Here's the drawing with two shaded views (mm, measured from the low corner). I have some questions. A direction names the side the tool comes from. Give positions to 0.01 mm unless a question says otherwise; leave off trailing zeros. Write each loop counter-clockwise with the first axis right and the second up, starting at its lowest first coordinate (ties: lowest second). Pieces come first, ordered by that corner, then holes. Notation, with made-up numbers: (58.5, -6.75) -> (100.5, -6.75) arc R26 cw to (100.5, 13.25) -> close; hole circle Ø7 at (31, 10). An arc over 180 degrees is marked (long way). One line per item, written item: value.
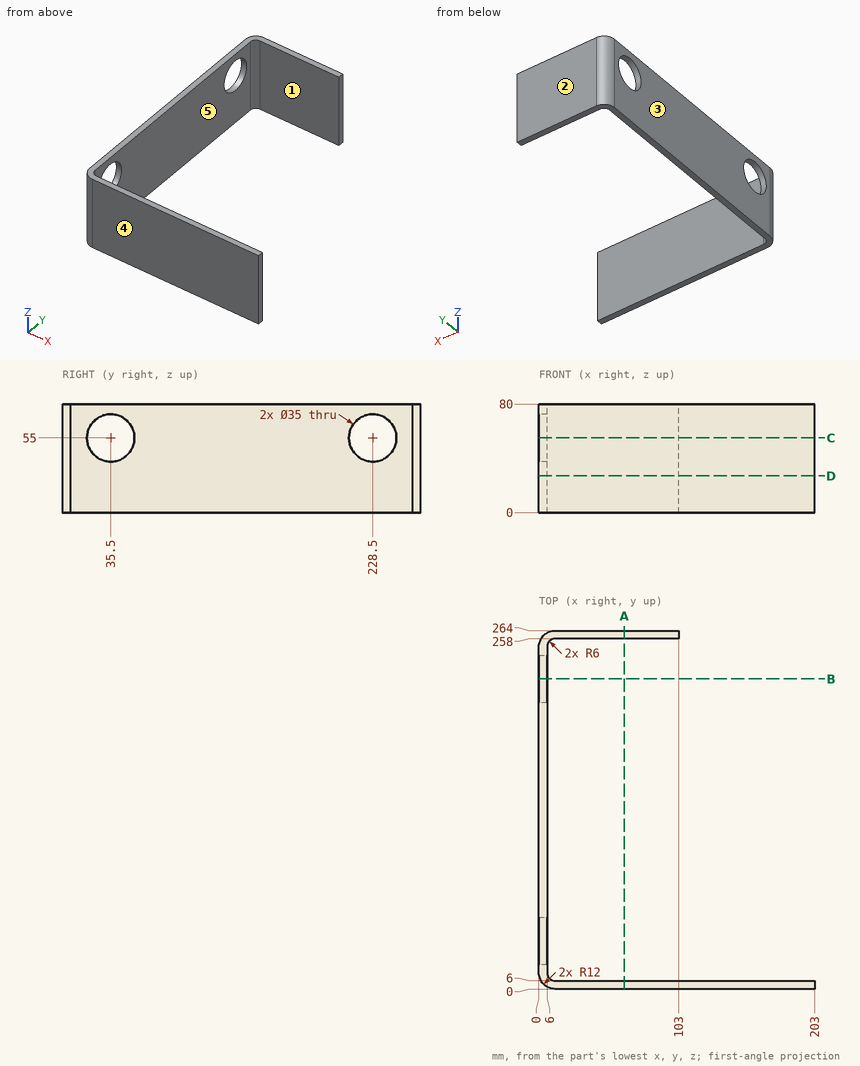
1) If we section it at A-A (x = 63): Write out the boundary of the cut face in (y, z), and give its area (3 significant figures).
Answer list:
outline: (0, 0) -> (6, 0) -> (6, 80) -> (0, 80) -> close; (258, 0) -> (264, 0) -> (264, 80) -> (258, 80) -> close
area: 960 mm^2
2) If we section it at B-B (y = 228.5): Write out the boundary of the cut face in (x, z).
Answer list:
outline: (0, 0) -> (6, 0) -> (6, 37.5) -> (0, 37.5) -> close; (0, 72.5) -> (6, 72.5) -> (6, 80) -> (0, 80) -> close
3) If we section it at C-C (z = 55): Write out the boundary of the cut face in (x, y).
Answer list:
outline: (0, 12) arc R12 ccw to (12, 0) -> (203, 0) -> (203, 6) -> (12, 6) arc R6 cw to (6, 12) -> (6, 18) -> (0, 18) -> close; (0, 53) -> (6, 53) -> (6, 211) -> (0, 211) -> close; (0, 246) -> (6, 246) -> (6, 252) arc R6 cw to (12, 258) -> (103, 258) -> (103, 264) -> (12, 264) arc R12 ccw to (0, 252) -> close
4) We'd pull the mould along Y, two halves only. Please class the marked faces 3, 4 and 5: released by +Y, released by -Y, zero draft, split by the parting line, or undercut.
Answer list:
face 3: zero draft
face 4: released by -Y
face 5: undercut
5) For the marked faces 1 and 2, which set-ups out of +Z, -Z, +X, -X, +Y, -Y let a thin tool reach every point of the face, with its end or its side?
Answer list:
face 1: +Z, -Z, +X
face 2: +Z, -Z, +X, -X, +Y
6) If we section it at D-D (z = 27): Write out the boundary of the cut face in (x, y), and give its area (3 significant figures).
Answer list:
outline: (0, 12) arc R12 ccw to (12, 0) -> (203, 0) -> (203, 6) -> (12, 6) arc R6 cw to (6, 12) -> (6, 252) arc R6 cw to (12, 258) -> (103, 258) -> (103, 264) -> (12, 264) arc R12 ccw to (0, 252) -> close
area: 3,300 mm^2
7) Will these pins go through, and if not, where does the flat tip stop? pin 1 (2 mm diameter, centred on y = 203, z = 31, fed in from +X); pin 2 (3 mm diameter, centred on y = 260.5, z = 55, fed in from +X).
Answer list:
pin 1: stops at x = 6
pin 2: stops at x = 103
8) I need wall thicknesses on L1, parallel to Y at x = 37.5, z = 60.5; L2, parallel to Y at x = 2.45, z = 55; L3, parallel to Y at x = 4.75, z = 55. Which ranges of each line are inside material? Lowest first, please.
Answer list:
L1: y = 0 to 6, 258 to 264
L2: y = 4.73 to 18, 53 to 211, 246 to 259.27
L3: y = 2.44 to 18, 53 to 211, 246 to 261.56
